from build123d import *

# Parameters (mm, degrees)
F0_W     = 12
F0_H     = 23
F1_DEPTH = 23
F3_DEPTH = 4
F4_W     = 12
F4_H     = 2.2
F5_DEPTH = 5
F6_DEPTH = 28
F8_DEPTH = 4.36513


with BuildPart() as f1:
    # F0 (on Front) → F1 (new body)
    with BuildSketch(Plane.XZ):
        with Locations((6, -11.5)):
            Rectangle(F0_W, F0_H)
    extrude(amount=F1_DEPTH)

    # F2 (on face) → F3 (join)
    with BuildSketch(Plane.XZ.offset(23)):
        with BuildLine():
            ThreePointArc((3.556097, -11.79521), (6, -11.25), (8.443903, -11.79521))
            ThreePointArc((8.443903, -11.79521), (8.67238, -11.183078), (8.75, -10.534323))
            ThreePointArc((8.75, -10.534323), (5.351245, -7.861942), (3.556097, -11.79521))
        make_face()
        with BuildLine():
            ThreePointArc((3.556097, -11.79521), (6, -13.284323), (8.443903, -11.79521))
            ThreePointArc((8.443903, -11.79521), (6, -11.25), (3.556097, -11.79521))
        make_face()
        with BuildLine():
            ThreePointArc((3.556097, -11.79521), (2.916977, -21.853604), (11.75, -17))
            ThreePointArc((11.75, -17), (10.853604, -13.916977), (8.443903, -11.79521))
            ThreePointArc((8.443903, -11.79521), (6, -13.284323), (3.556097, -11.79521))
        make_face()
    extrude(amount=F3_DEPTH)

    # F4 (on face) → F5 (join)
    with BuildSketch(Plane.XY):
        with Locations((6, -17.1)):
            Rectangle(F4_W, F4_H)
    extrude(amount=F5_DEPTH)

    # F4 (on face) → F6 (join)
    with BuildSketch(Plane.XY):
        with Locations((6, -17.1)):
            Rectangle(F4_W, F4_H)
    extrude(amount=-F6_DEPTH)

    # F7 (on face) → F8 (cut)
    with BuildSketch(Plane.XZ.offset(18.2)):
        with BuildLine():
            Line((6.998493, -29.572871), (6.998493, -26.675947))
            Line((6.998493, -26.675947), (6.998493, -26.566196))
            ThreePointArc((6.998493, -26.566196), (5.96604, -25.621648), (5.000085, -26.634102))
            Line((5.000085, -26.634102), (5.036416, -29.422127))
            Line((5.036416, -29.422127), (6.998493, -29.572871))
        make_face()
    extrude(amount=-F8_DEPTH, mode=Mode.SUBTRACT)


solid = f1.part
Can you work these out from the model? Positions are in its coordinate system, mm. A direction names the side the tool comes from. Coordinates: 2 decimals unless noted, no trailing zeros. Write each loop counter-clockwise with the first axis right and the second up, starting at its lowest first coordinate (ties: lowest second). Pieces come first, ordered by that corner, then holes. Notation, with made-up numbers: (-6, 84.5) -> (30, 84.5) arc R14 ccw to (30, 108.5) -> close; hole circle Ø2 at (9, 83). An arc over 180 degrees is marked (long way). Answer as CSV lines item,"result".
1) If we section it at B-B on z = -2: Please give me the cut outline in (x, y).
Check result:
outline,"(0, -23) -> (12, -23) -> (12, 0) -> (0, 0) -> close"
2) If we mould it in two halves opening along X, with no side actions, what happens to faces 5 (the flat face through (12, -11, -12)), 6 (the flat face through (6.998, -17, -27)), 7 (the flat face through (6, -8, 0))? For each: +X half, -X half, draft (parallel to the pull), parting line (faces both ways), or undercut.
Check result:
face 5,"+X half"
face 6,"undercut"
face 7,"draft"
3) If we section it at A-A on x = 6: Please give me the cut outline in (y, z), then the cut area to 3 significant figures.
Check result:
outline,"(-27, -22.75) -> (-23, -22.75) -> (-23, -23) -> (-18.2, -23) -> (-18.2, -25.62) -> (-16, -25.62) -> (-16, -23) -> (0, -23) -> (0, 0) -> (-16, 0) -> (-16, 5) -> (-18.2, 5) -> (-18.2, 0) -> (-23, 0) -> (-23, -7.78) -> (-27, -7.78) -> close"
area,"606 mm²"
4) Will these pins go through, and if not, where does the flat tip stop? P1, Ø2.5, axis at x = 4.5, z = -24.5, coming from the +Y side; P2, Ø2.5, axis at x = 4, y = -20.5, coming from the +Z side; P3, Ø2.5, axis at x = 3.5, z = -26, coming from the -Y side.
Check result:
P1,"y = -16"
P2,"z = 0"
P3,"y = -18.2"
5) If I drill on line 1 (Y direction, x = 2.25, z = -11); line 2 (Y direction, x = 5, z = -24.5), over which ranges is the centre line in solid material (lowest first)? Write a range as from..to.
Check result:
line 1,"-23..0"
line 2,"-18.2..-16"
6) On a 3-axis mill with a long thin cutter (end or side, diameter ignored), from which of +Z, -Z, +X, -X, +Y, -Y can I reach the whole of each face in a straight line? I mean faces 1 (the flat face through (6, -18.2, 2)), 2 (the flat face through (6, -16, 2)), 3 (the flat face through (6, -18.2, -25)), 4 (the flat face through (6, -8, -23)). Say none if no direction works.
Check result:
face 1,"+Z, +X, -X, -Y"
face 2,"+Z, +X, -X, +Y"
face 3,"-Z, +X, -X, -Y"
face 4,"-Z, +X, -X, +Y"
7) If we section it at D-D on x = 10.5: Please give me the cut outline in (y, z), then the cut area to 3 significant figures.
Check result:
outline,"(-27, -20.58) -> (-23, -20.58) -> (-23, -23) -> (-18.2, -23) -> (-18.2, -28) -> (-16, -28) -> (-16, -23) -> (0, -23) -> (0, 0) -> (-16, 0) -> (-16, 5) -> (-18.2, 5) -> (-18.2, 0) -> (-23, 0) -> (-23, -13.42) -> (-27, -13.42) -> close"
area,"580 mm²"
